Read the model definition and answer for the solid it produces. Units are mm, in the model's axes. A direction names the side the tool comes from. Coordinates: 2 decimals unless noted, no trailing zeros. Loops run counter-clockwise (first coordinate to the right, second up) from the corner with the lowest first, then second, coordinate; pieces in that order, holes last. Notation, with made-up numbers: (2.5, -16.75) -> (24.5, -16.75) arc R22 cw to (24.5, 15.25) -> close; hole circle Ø2 at (-18.75, 59). An arc over 180 degrees is marked (long way). Answer in a Markdown table with one row per item.
```python
from build123d import *

# Parameters (mm, degrees)
SKETCH2_R           = 7.9375
SKETCH2_R_2         = 6.35
BOSS_EXTRUDE1_DEPTH = 12.7


with BuildPart() as part:
    # Sketch2 → Boss-Extrude1 (new body)
    with BuildSketch(Plane.XY):
        with BuildLine():
            Line((-28.210760469, -18.251004821), (-10.08654579, -0.126790143))
            Line((-10.08654579, -0.126790143), (-28.210760469, 17.997424536))
            ThreePointArc((-28.210760469, 17.997424536), (-35.394965366, 35.341629433), (-18.050760469, 28.157424536))
            Line((-18.050760469, 28.157424536), (0.07345421, 10.033209857))
            Line((0.07345421, 10.033209857), (18.197668889, 28.157424536))
            ThreePointArc((18.197668889, 28.157424536), (35.541873785, 35.341629433), (28.357668889, 17.997424536))
            Line((28.357668889, 17.997424536), (10.23345421, -0.126790143))
            Line((10.23345421, -0.126790143), (28.357668889, -18.251004821))
            ThreePointArc((28.357668889, -18.251004821), (35.541873785, -35.595209718), (18.197668889, -28.411004821))
            Line((18.197668889, -28.411004821), (0.07345421, -10.286790143))
            Line((0.07345421, -10.286790143), (-18.050760469, -28.411004821))
            ThreePointArc((-18.050760469, -28.411004821), (-35.394965366, -35.595209718), (-28.210760469, -18.251004821))
        make_face()
        with Locations((-28.210760469, 28.157424536)):
            Circle(SKETCH2_R, mode=Mode.SUBTRACT)
        with Locations((28.357668889, 28.157424536)):
            Circle(SKETCH2_R, mode=Mode.SUBTRACT)
        with Locations((28.357668889, -28.411004821)):
            Circle(SKETCH2_R, mode=Mode.SUBTRACT)
        with Locations((-28.210760469, -28.411004821)):
            Circle(SKETCH2_R, mode=Mode.SUBTRACT)
        with Locations((0.07345421, -0.126790143)):
            Circle(SKETCH2_R_2, mode=Mode.SUBTRACT)
    extrude(amount=BOSS_EXTRUDE1_DEPTH)


solid = part.part
```
1. A tool of negligible diameter and unlimited length cuts with its end or side. For faces 5 (the cylindrical face through (-35.15, -35.83, 6.26)), 6 (the flat face through (19.169, -9.062, 6.261)), 7 (the flat face through (-9.116, 19.222, 6.261)), 8 (the flat face through (-8.86, -19.22, 6.26)), from which of +Z, -Z, +X, -X, +Y, -Y can it reach the whole face along a straight path? Write none if from no direction.
A:
| item | result |
|---|---|
| face 5 | +Z, -Z |
| face 6 | +Z, -Z, +X |
| face 7 | +Z, -Z, +Y |
| face 8 | +Z, -Z, -Y |
2. A cutting plane is placed at C-C on x = 15. Give the vertices of the cut face in (y, z).
A:
| item | result |
|---|---|
| outline | (-25.21, 0) -> (-4.89, 0) -> (-4.89, 12.7) -> (-25.21, 12.7) -> close; (4.64, 0) -> (24.96, 0) -> (24.96, 12.7) -> (4.64, 12.7) -> close |
3. A cutting plane is placed at A-A on z = 7.5. Count the separate pieces of the cut face and the enclosed holes in it, and give its area (3 significant figures).
A:
| item | result |
|---|---|
| separate pieces | 1 |
| enclosed holes | 5 |
| area | 1,940 mm2 |
4. A cutting plane is placed at B-B on y = -24. Give the vertices of the cut face in (x, z), and give its area (3 significant figures).
A:
| item | result |
|---|---|
| outline | (-37.36, 0) -> (-34.81, 0) -> (-34.81, 12.7) -> (-37.36, 12.7) -> close; (-21.61, 0) -> (-13.64, 0) -> (-13.64, 12.7) -> (-21.61, 12.7) -> close; (13.79, 0) -> (21.76, 0) -> (21.76, 12.7) -> (13.79, 12.7) -> close; (34.96, 0) -> (37.51, 0) -> (37.51, 12.7) -> (34.96, 12.7) -> close |
| area | 267 mm2 |
5. The mould has two halves that part along Y. Classify faces 1 (the cylindrical face through (20.428, -28.062, 6.261)), 2 (the flat face through (9.262, -19.476, 6.261)), 3 (the flat face through (-19.28, -9.32, 6.26)), 4 (the flat face through (9.01, 18.97, 6.26)): pulls with the +Y half, pulls with the -Y half, needs draft (parallel to the pull), parting line crosses it, or undercut.
A:
| item | result |
|---|---|
| face 1 | undercut |
| face 2 | pulls with the -Y half |
| face 3 | undercut |
| face 4 | pulls with the +Y half |
6. A cutting plane is placed at D-D on x = 23. Give the vertices of the cut face in (y, z), and give its area (3 significant figures).
A:
| item | result |
|---|---|
| outline | (-37.04, 0) -> (-34.27, 0) -> (-34.27, 12.7) -> (-37.04, 12.7) -> close; (-22.55, 0) -> (-12.89, 0) -> (-12.89, 12.7) -> (-22.55, 12.7) -> close; (12.64, 0) -> (22.3, 0) -> (22.3, 12.7) -> (12.64, 12.7) -> close; (34.01, 0) -> (36.79, 0) -> (36.79, 12.7) -> (34.01, 12.7) -> close |
| area | 316 mm2 |
7. Given pin 1 Ø4 at (y, z) = (-17.5, 10) entering from -X; pin 2 Ø2 at (x, z) = (-2, 9) entering from +Y, each flat-ended and moving along its own axis, determine where each tip first touches the part or whether it passes through.
A:
| item | result |
|---|---|
| pin 1 | stops at x = -33.09 |
| pin 2 | stops at y = 13.11 |
8. Find the intervals of material crossed by probe 1 along Y at (x, z) = (-25, 8.5); probe 2 along Y at (x, z) = (-28.5, 2.75); probe 3 along X at (y, z) = (35, 2.25), in increasing order.
A:
| item | result |
|---|---|
| probe 1 | y = -38.05 to -35.67, -21.15 to -15.04, 14.79 to 20.9, 35.42 to 37.8 |
| probe 2 | y = -38.57 to -36.34, -20.48 to -18.26, 18 to 20.23, 36.09 to 38.31 |
| probe 3 | x = -35.72 to -32.23, -24.19 to -20.7, 20.85 to 24.33, 32.38 to 35.87 |
